```python
from build123d import *

# Parameters (mm, degrees)
SKETCH1_W           = 20
SKETCH1_H           = 60
BOSS_EXTRUDE1_DEPTH = 30
SKETCH2_W           = 40
SKETCH2_H           = 40
BOSS_EXTRUDE2_DEPTH = 20
FILLET1_R           = 10


with BuildPart() as part:
    # Sketch1 → Boss-Extrude1 (new body)
    with BuildSketch(Plane.XY):
        with Locations((-20, -30)):
            Rectangle(SKETCH1_W, SKETCH1_H)
    extrude(amount=BOSS_EXTRUDE1_DEPTH)

    # Sketch2 → Boss-Extrude2 (add)
    with BuildSketch(Plane.XY):
        with Locations((-10, -40)):
            Rectangle(SKETCH2_W, SKETCH2_H)
    extrude(amount=-BOSS_EXTRUDE2_DEPTH)

    # Fillet1
    fillet1_edges = [part.edges().sort_by_distance(p)[0] for p in [
        (10, -20, -10),
        (-20, 0, 30),
    ]]
    fillet(fillet1_edges, radius=FILLET1_R)


solid = part.part
```
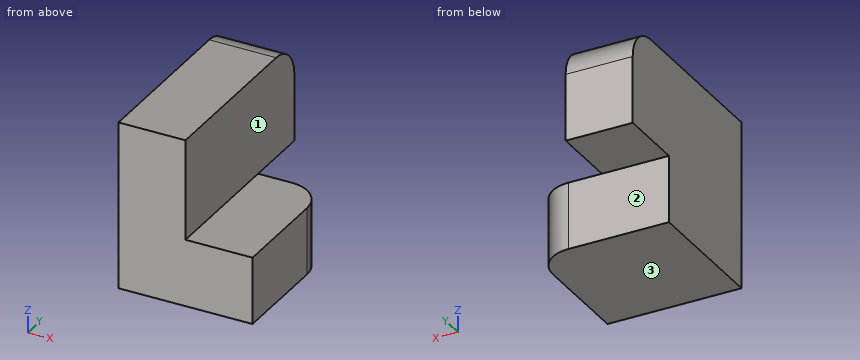
Could you check a few things on this model? Use its own coordinates, in mm. Face numbers are marked on the shaded views. A direction names the side the tool comes from. Coordinates: 2 decimals unless noted, no trailing zeros. Write each loop counter-clockwise with the first axis right and the second up, starting at its lowest first coordinate (ties: lowest second). Pieces come first, ordered by that corner, then holes. Notation, with made-up numbers: M -16,30 L 2,30 A16 cw 2,37 Z; hole C 17.5,71.25 d9. An arc over 180 degrees is marked long. Answer as CSV lines item,"result". Start each with the question number.
1) I want a section at B-B, the plane y = -48.5. Please give me the cut outline in (x, z).
2) I want a section at C-C, the plane z = -3.5. Please give me the cut outline in (x, y).
3) I want a section at A-A, the plane x = -14. Please give me the cut outline in (y, z), and give its area (3 significant figures).
4) I want a section at D-D, the plane x = -5.5. Please give me the cut outline in (y, z), and give its area (3 significant figures).
5) For P1, Ø8, axis at x = -7.5, y = -48.5, coming from the +Z side; P2, Ø6, axis at x = 4.5, y = -43, coming from the +Z side; P3, Ø10, axis at y = -17, z = 13, coming from the +X side; P4, Ø10, axis at x = -20.5, y = -8, coming from the -Z side, each with a flat end and sliding along its axis, tell me the tip position at first contact or that it passes through.
6) For the marked faces 1, 2 and 3, which set-ups out of +Z, -Z, +X, -X, +Y, -Y let a thin tool reach every point of the face, with its end or its side?
7) Please list where these lines run through material, in increasing order: line 1 (Z direction, x = -25.5, y = -14); line 2 (Z direction, x = -9, y = -36); line 3 (X direction, y = -26, z = 13). Write a range as from..to.
Data:
1,outline,"M -30,-20 L 10,-20 L 10,0 L -10,0 L -10,30 L -30,30 Z"
2,outline,"M -30,-60 L 10,-60 L 10,-30 A10 ccw 0,-20 L -30,-20 Z"
3,outline,"M -60,-20 L -20,-20 L -20,0 L 0,0 L 0,20 A10 ccw -10,30 L -60,30 Z"
3,area,"2,580 mm^2"
4,outline,"M -60,-20 L -20,-20 L -20,0 L -60,0 Z"
4,area,"800 mm^2"
5,P1,"stops at z = 30"
5,P2,"stops at z = 0"
5,P3,"stops at x = -10"
5,P4,"stops at z = 0"
6,face 1,"+Z, +X, +Y, -Y"
6,face 2,"-Z, +X, -X, +Y"
6,face 3,"-Z, +X, -X, +Y, -Y"
7,line 1,"z = 0..30"
7,line 2,"z = -20..0"
7,line 3,"x = -30..-10"
